Check sheet for the modelled part. Datum: model origin and axes. Units: mm. A direction names the side the tool comes from. Give positions to 0.01 mm unless a question says otherwise; leave off trailing zeros. Order: outer loops, then holes, each group sorted by start corner. A loop starts at its lowest first (then second) coordinate and runs counter-clockwise, first axis right, second up.
```python
from build123d import *

# Parameters (mm, degrees)
SKETCH_1_W          = 10
SKETCH_1_H          = 3
EXTRUDE_1_DEPTH     = 10
SKETCH_2_R          = 3.3
CUT_EXTRUDE_1_DEPTH = 11
SKETCH_3_R          = 1.75
CUT_EXTRUDE_2_DEPTH = 4
FILLET_1_R          = 3
FILLET_2_R          = 1


with BuildPart() as part:
    # ｽｹｯﾁ1 → ﾎﾞｽ - 押し出し1 (new body)
    with BuildSketch(Plane.XY):
        Polygon((5, 10), (0, 10), (0, -5), (5, -5), (5, 7), align=None)
        with Locations((10, 8.5)):
            Rectangle(SKETCH_1_W, SKETCH_1_H)
        Polygon((0, -5), (0, 10), (-5, 10), (-5, 7), (-5, -5), align=None)
        with Locations((-10, 8.5)):
            Rectangle(SKETCH_1_W, SKETCH_1_H)
    extrude(amount=EXTRUDE_1_DEPTH)

    # ｽｹｯﾁ2 → ｶｯﾄ - 押し出し1 (cut, through all)
    with BuildSketch(Plane(origin=(0, 0, 0), x_dir=(-1, 0, 0), z_dir=(0, 0, -1))):
        Circle(SKETCH_2_R)
    extrude(amount=-CUT_EXTRUDE_1_DEPTH, mode=Mode.SUBTRACT)

    # ｽｹｯﾁ3 → ｶｯﾄ - 押し出し2 (cut, through all)
    with BuildSketch(Plane.XZ.offset(-7)):
        with Locations((-11.5, 5)):
            Circle(SKETCH_3_R)
        with Locations((11.5, 5)):
            Circle(SKETCH_3_R)
    extrude(amount=-CUT_EXTRUDE_2_DEPTH, mode=Mode.SUBTRACT)

    # ﾌｨﾚｯﾄ1
    fillet_1_edges = [part.edges().sort_by_distance(p)[0] for p in [
        (5, -5, 5),
        (-5, -5, 5),
        (-5, 7, 5),
        (5, 7, 5),
    ]]
    fillet(fillet_1_edges, radius=FILLET_1_R)

    # ﾌｨﾚｯﾄ2
    fillet_2_edges = [part.edges().sort_by_distance(p)[0] for p in [
        (-15, 8.5, 0),
        (15, 8.5, 0),
        (15, 8.5, 10),
        (-15, 7, 5),
        (15, 7, 5),
        (-15, 8.5, 10),
        (-5, 1, 0),
        (-5, 1, 10),
        (-11.5, 7, 0),
        (-11.5, 7, 10),
        (11.5, 7, 0),
        (11.5, 7, 10),
        (5, 1, 0),
        (5, 1, 10),
        (0, -5, 0),
        (0, -5, 10),
        (4.121320344, -4.121320344, 0),
        (-4.121320344, -4.121320344, 0),
        (4.121320344, -4.121320344, 10),
        (-4.121320344, -4.121320344, 10),
        (-5.878679656, 6.121320344, 0),
        (-5.878679656, 6.121320344, 10),
        (5.878679656, 6.121320344, 0),
        (5.878679656, 6.121320344, 10),
    ]]
    fillet(fillet_2_edges, radius=FILLET_2_R)


solid = part.part
```
(1) Thickness scan on L1, parallel to Z at x = -11.5, y = 9.1; L2, parallel to X at y = 9.25, z = 3.5; L3, parallel to X at y = 9, z = 5.25. Record the ranges inside material, lowest first.
(2) Sectioned sample at A-A (y = 0). Enter the section's corners in (x, z), plus the area to 3 significant figures.
(3) Release check for a two-part mould opening along Z. For faces 1 (the face through (-10.958, 7.301, 0.285)), 2 (the face through (12.31, 8.48, 3.45)), 3 (the face through (-4.699, 0.958, 9.715)) record: released by +Z, released by -Z, zero draft, split by the parting line, or undercut.
(4) Sectioned sample at D-D (z = 1.75). Enter the section's corners in (x, y).
(5) Sectioned sample at C-C (x = 11.5). Enter the section's corners in (y, z), plus the area to 3 significant figures.
(6) Go/stop test with flat-tipped pins: P1, Ø8, axis at x = -2.5, y = 4, coming from the -Z side; P2, Ø3, axis at y = 0, z = 4.5, coming from the +X side; P3, Ø5, axis at y = 1.5, z = 4, coming from the -X side; P4, Ø6, axis at x = -8.5, z = 6.5, coming from the -Y side. Record where each tip stops, or that it passes through.
(7) Tool access check on faces 4 (the face through (9.6, 7, 4.9)), 5 (the face through (4.699, 1.042, 9.715)), 6 (the face through (11.042, 7.301, 0.285)), 7 (the face through (-9.7, 7, 4.1)). Record the directions out of +Z, -Z, +X, -X, +Y, -Y that give a thin tool (end or side, any length) a straight path to the whole face; none if there is none.
(8) Sectioned sample at B-B (z = 4.5). Enter the section's corners in (x, y), plus the area to 3 significant figures.
Values follow:
1. L1: z = 0 to 3.25, 6.75 to 10
1. L2: x = -15 to -12.4, -10.6 to 10.6, 12.4 to 15
1. L3: x = -15 to -13.23, -9.77 to 9.77, 13.23 to 15
2. outline: (-5, 1) arc R1 ccw to (-4, 0) - (-3.3, 0) - (-3.3, 10) - (-4, 10) arc R1 ccw to (-5, 9) - close; (3.3, 0) - (4, 0) arc R1 ccw to (5, 1) - (5, 9) arc R1 ccw to (4, 10) - (3.3, 10) - close
2. area: 33.1 mm2
3. face 1: released by -Z
3. face 2: undercut
3. face 3: released by +Z
4. outline: (-15, 8) arc R1 ccw to (-14, 7) - (-8, 7) arc R3 cw to (-5, 4) - (-5, -2) arc R3 ccw to (-2, -5) - (2, -5) arc R3 ccw to (5, -2) - (5, 4) arc R3 cw to (8, 7) - (14, 7) arc R1 ccw to (15, 8) - (15, 10) - (-15, 10) - close; hole circle Ø6.6 at (0, 0)
5. outline: (7, 1) arc R1 ccw to (8, 0) - (10, 0) - (10, 3.25) - (7, 3.25) - close; (7, 6.75) - (10, 6.75) - (10, 10) - (8, 10) arc R1 ccw to (7, 9) - close
5. area: 19.1 mm2
6. P1: stops at z = 0
6. P2: stops at x = 5
6. P3: stops at x = -5
6. P4: stops at y = 5.66
7. face 4: +Z, -Z, +X, -Y
7. face 5: +Z, +X, -Y
7. face 6: -Z, +X, -Y
7. face 7: +Z, -Z, -X, -Y
8. outline: (-15, 8) arc R1 ccw to (-14, 7) - (-13.18, 7) - (-13.18, 10) - (-15, 10) - close; (-9.82, 7) - (-8, 7) arc R3 cw to (-5, 4) - (-5, -2) arc R3 ccw to (-2, -5) - (2, -5) arc R3 ccw to (5, -2) - (5, 4) arc R3 cw to (8, 7) - (9.82, 7) - (9.82, 10) - (-9.82, 10) - close; (13.18, 7) - (14, 7) arc R1 ccw to (15, 8) - (15, 10) - (13.18, 10) - close; hole circle Ø6.6 at (0, 0)
8. area: 155 mm2
